```python
from build123d import *

# Parameters (mm, degrees)
F0_W     = 200
F0_H     = 200
F1_DEPTH = 9
F2_R     = 2.983791
F2_R_2   = 2.5
F3_DEPTH = 25
F4_DEPTH = 15


with BuildPart() as f1:
    # F0 (on Top) → F1 (new body)
    with BuildSketch(Plane.XY):
        Rectangle(F0_W, F0_H)
    extrude(amount=F1_DEPTH)

    # F2 (on face) → F3 (cut)
    with BuildSketch(Plane.YZ.offset(100)):
        with Locations((-50, 4.5)):
            Circle(F2_R)
        with Locations((50, 4.5)):
            Circle(F2_R_2)
    extrude(amount=-F3_DEPTH, mode=Mode.SUBTRACT)

    # F2 (on face) → F4 (cut)
    with BuildSketch(Plane.YZ.offset(100)):
        with Locations((-50, 4.5)):
            Circle(F2_R)
    extrude(amount=-F4_DEPTH, mode=Mode.SUBTRACT)


solid = f1.part
```
Build history of the part. All positions in model axes, mm. A direction names the side the tool comes from. Round coordinates to 2 decimals unless told otherwise and drop trailing zeros. Order: outer loops, then holes, each group sorted by start corner. A loop starts at its lowest first (then second) coordinate and runs counter-clockwise, first axis right, second up. Notation, with made-up numbers: (54.5, 65.5) -> (69.5, 65.5) arc R25 ccw to (69.5, 104.5) -> close; hole circle Ø8 at (25.25, 2). An arc over 180 degrees is marked (long way). Answer in a Markdown table with one row per item.
1) Pin check, flat tips, straight feed: P1, Ø4, axis at y = -51.5, z = 3, coming from the +X side; P2, Ø4, axis at y = 50, z = 4.5, coming from the +X side. Stop position of each tip, or through.
Values:
| item | result |
|---|---|
| P1 | x = 100 |
| P2 | x = 75 |
2) Mould opens along Y. For faces 1 (the flat face through (100, -1, 4)), 2 (the flat face through (-1, -100, 4)), 3 (the cylindrical face through (87.68, 52.31, 3.54)) say: released by +Y, released by -Y, zero draft, split by the parting line, or undercut.
Values:
| item | result |
|---|---|
| face 1 | zero draft |
| face 2 | released by -Y |
| face 3 | undercut |
3) Band-saw the part on C-C on y = -50. Give the cut face in (x, z).
Values:
| item | result |
|---|---|
| outline | (-100, 0) -> (100, 0) -> (100, 1.52) -> (75, 1.52) -> (75, 7.48) -> (100, 7.48) -> (100, 9) -> (-100, 9) -> close |
4) Band-saw the part on B-B on y = 50. Give the cut face in (x, z).
Values:
| item | result |
|---|---|
| outline | (-100, 0) -> (100, 0) -> (100, 2) -> (75, 2) -> (75, 7) -> (100, 7) -> (100, 9) -> (-100, 9) -> close |
5) Band-saw the part on A-A on x = 79.5. Give the cut face in (y, z).
Values:
| item | result |
|---|---|
| outline | (-100, 0) -> (100, 0) -> (100, 9) -> (-100, 9) -> close; hole circle Ø5.97 at (-50, 4.5); hole circle Ø5 at (50, 4.5) |
6) Which spindle directions (+Z, -Z, +X, -X, +Y, -Y) get a long thin tool onto all of the face, cutting with end or side? Do faces 4 (the flat face through (75, 50, 5)), 5 (the flat face through (-1, 1, 9)). Say none if no direction does.
Values:
| item | result |
|---|---|
| face 4 | +X |
| face 5 | +Z, +X, -X, +Y, -Y |
7) Wall check: L1, parallel to Y at x = 79.5, z = 4; L2, parallel to Z at x = 87.5, y = -50; L3, parallel to Z at x = 94.75, y = 50. Give the ranges that are in metal, low to high.
Values:
| item | result |
|---|---|
| L1 | -100 to -52.94, -47.06 to 47.55, 52.45 to 100 |
| L2 | 0 to 1.52, 7.48 to 9 |
| L3 | 0 to 2, 7 to 9 |
